Work out the finished part from the listing and answer in its coordinate system (mm). A direction names the side the tool comes from. Round coordinates to 2 decimals unless told otherwise and drop trailing zeros. Order: outer loops, then holes, each group sorted by start corner. A loop starts at its lowest first (then second) coordinate and runs counter-clockwise, first axis right, second up. Notation, with made-up numbers: (68, 7) - (92, 7) arc R31 cw to (92, 32) - close; hole circle Ø9 at (-12.75, 34.5). An arc over 180 degrees is marked (long way). Use one line per item in the form item = value. Start each with the question number.
Q1. Given P1, Ø1.5, axis at y = -5, z = 16.5, coming from the -X side; P2, Ø1.9, axis at x = -72, y = 8.5, coming from the +Z side; P3, Ø1.9, axis at x = -72, y = -18.5, coming from the +Z side; P4, Ø1, axis at x = 72.5, z = 44.5, coming from the +Y side, each flat-ended and moving along its own axis, determine where each tip first touches the part or whether it passes through.
Q2. The part is cut by section D-D on x = 7. Determine the outline of the cut face in (y, z).
Q3. The part is cut by section C-C on z = 16.5. Determine the outline of the cut face in (x, y), plus the area to 3 significant figures.
Q4. The part is cut by section A-A on z = 47. Determine the outline of the cut face in (x, y).
Q5. Which of the six approach directions +Z, -Z, +X, -X, +Y, -Y give full straight-line access (tool end or side, diameter ignored) to faces 3 (the flat face through (-73, -25.4, 3)), 4 (the flat face through (-73, 9, 5.8)), 5 (the flat face through (-73, -16, 6.367))?
Q6. For a pull along X with two mould halves and no side action, classify faces 1 (the cylindrical face through (11.026, -3.131, 85.988)), 2 (the flat face through (-73, 19.05, 3)) as +X half, -X half, draft (parallel to the pull), parting line (faces both ways), or undercut.
Q7. Find the intervals of material crossed by line 1 (Y direction, x = -50, z = 57); line 2 (Z direction, x = -46.5, y = -3), in increasing order. Write a range as [from, to].
from build123d import *

# Parameters (mm, degrees)
F1_DEPTH = 6.35
F3_DEPTH = 19.05
F5_DEPTH = 19.05


with BuildPart() as f1:
    # F0 (on Front) → F1 (new body)
    with BuildSketch(Plane.XZ):
        with BuildLine():
            ThreePointArc((-70.237749294, 0), (9.137250706, 79.375), (88.512250706, 0))
            Line((88.512250706, 0), (94.862250706, 0))
            ThreePointArc((94.862250706, 0), (9.137250706, 86.0083166132), (-76.587749294, 0))
            Line((-76.587749294, 0), (-70.237749294, 0))
        make_face()
    extrude(amount=F1_DEPTH)

    # F2 (on face) → F3 (join)
    with BuildSketch(Plane.XZ.offset(6.35)):
        with BuildLine():
            Line((-76.587749294, 0), (-70.237749294, 0))
            ThreePointArc((-70.237749294, 0), (-70.1737860692, 3.1859175505), (-69.9819994827, 6.3667004474))
            Line((-69.9819994827, 6.3667004474), (-76.3720610245, 6.3667004474))
            Line((-76.3720610245, 6.3667004474), (-76.587749294, 0))
        make_face()
    extrude(amount=F3_DEPTH)

    # F4 (on face) → F5 (join)
    with BuildSketch(Plane(origin=(0, 0, 0), x_dir=(-1, 0, 0), z_dir=(0, 1, 0))):
        with BuildLine():
            ThreePointArc((70.0255849548, 5.7996616405), (70.1846904754, 2.9017705307), (70.237749294, 0))
            Line((70.237749294, 0), (76.587749294, 0))
            Line((76.587749294, 0), (76.4105161745, 5.7996616405))
            Line((76.4105161745, 5.7996616405), (70.0255849548, 5.7996616405))
        make_face()
    extrude(amount=F5_DEPTH)


solid = f1.part
Found:
q1.P1 = -75.18
q1.P2 = 5.8
q1.P3 = 6.37
q1.P4 = through
q2.outline = (-6.35, 79.35) - (0, 79.35) - (0, 85.98) - (-6.35, 85.98) - close
q3.outline = (-75.04, -6.35) - (-68.5, -6.35) - (-68.5, 0) - (-75.04, 0) - close; (86.78, -6.35) - (93.31, -6.35) - (93.31, 0) - (86.78, 0) - close
q3.area = 83.0 mm²
q4.outline = (-62.74, -6.35) - (-54.83, -6.35) - (-54.83, 0) - (-62.74, 0) - close; (73.1, -6.35) - (81.01, -6.35) - (81.01, 0) - (73.1, 0) - close
q5.face_3 = +Z, -Z, +X, -X, -Y
q5.face_4 = +Z, +X, -X, +Y
q5.face_5 = +Z, +X, -X, -Y
q6.face_1 = parting line
q6.face_2 = draft
q7.line_1 = [-6.35, 0]
q7.line_2 = [56.61, 65.5]
